The model under review builds one solid part; all positions refer to its coordinate system, in mm. A direction names the side the tool comes from. Round coordinates to 2 decimals unless told otherwise and drop trailing zeros. Order: outer loops, then holes, each group sorted by start corner. A loop starts at its lowest first (then second) coordinate and runs counter-clockwise, first axis right, second up.
```python
from build123d import *

# Parameters (mm, degrees)
PERIMETER_DEPTH      = 4.124453
PERIMETER_DEPTH_BACK = 31
SKETCH2_W            = 95.636537696
SKETCH2_H            = 63.255720718
SKETCH2_W_2          = 91.636537696
SKETCH2_H_2          = 59.255720718
USB_HOLE_START       = -66.6
SKETCH4_W            = 13.571838798
SKETCH4_H            = 8.15289322
USB_HOLE_DEPTH       = 81
BOTTOM_START         = -31
SKETCH2_12_W         = 95.636537696
SKETCH2_12_H         = 63.255720718
BOTTOM_DEPTH         = 2
SKETCH4_6_W          = 6
SKETCH4_6_H          = 2.002355377
LOCKING_HOLE_DEPTH   = 152
FILLET1_R            = 3
STRAWS_START         = -31
SKETCH2_14_R         = 2.578463196
SKETCH2_14_R_2       = 1.375
SKETCH2_14_R_3       = 2.558752615
SKETCH2_14_R_4       = 1.372691975
SKETCH2_14_R_5       = 2.568645486
SKETCH2_14_R_6       = 1.384737696
SKETCH2_14_R_7       = 2.568443666
SKETCH2_14_R_8       = 1.388555099
STRAWS_DEPTH         = 15.415068015
CUT_EXTRUDE3_START   = -68
SKETCH2_16_R         = 1.375
SKETCH2_16_R_2       = 1.388555099
SKETCH2_16_R_3       = 1.384737696
SKETCH2_16_R_4       = 1.372691975
CUT_EXTRUDE3_DEPTH   = 68


with BuildPart() as part:
    # Sketch2 → Perimeter (new, two sides: drawn at the far end of the back side and taken through both)
    with BuildSketch(Plane.XY.offset(-PERIMETER_DEPTH_BACK)):
        with Locations((147.401306837, -96.227860359)):
            Rectangle(SKETCH2_W, SKETCH2_H)
        with Locations((147.401306837, -96.227860359)):
            Rectangle(SKETCH2_W_2, SKETCH2_H_2, mode=Mode.SUBTRACT)
    extrude(amount=PERIMETER_DEPTH + PERIMETER_DEPTH_BACK)

    # Sketch4 → USB_Hole (cut)
    with BuildSketch(Plane(origin=(0, 0, 0), x_dir=(1, 0, 0), z_dir=(0, 1, 0)).offset(USB_HOLE_START)):
        with Locations((179.410729964, 14.588485375)):
            Rectangle(SKETCH4_W, SKETCH4_H)
    extrude(amount=-USB_HOLE_DEPTH, mode=Mode.SUBTRACT)

    # Sketch2<12> → Bottom (add)
    with BuildSketch(Plane.XY.offset(BOTTOM_START)):
        with Locations((147.401306837, -96.227860359)):
            Rectangle(SKETCH2_12_W, SKETCH2_12_H)
    extrude(amount=-BOTTOM_DEPTH)

    # Sketch4<6> → Locking_Hole (cut)
    with BuildSketch(Plane(origin=(0, 0, 0), x_dir=(1, 0, 0), z_dir=(0, 1, 0))):
        with Locations((131.455, 4.874369651)):
            Rectangle(SKETCH4_6_W, SKETCH4_6_H)
        with Locations((183.452691975, 4.874369651)):
            Rectangle(SKETCH4_6_W, SKETCH4_6_H)
    extrude(amount=-LOCKING_HOLE_DEPTH, mode=Mode.SUBTRACT)

    # Fillet1
    fillet1_edges = [part.edges().sort_by_distance(p)[0] for p in [
        (101.583037989, -125.855720718, -13.4377735),
        (101.583037989, -66.6, -13.4377735),
        (193.219575685, -66.6, -13.4377735),
        (195.219575685, -64.6, -14.4377735),
        (193.219575685, -125.855720718, -13.4377735),
        (195.219575685, -127.855720718, -14.4377735),
        (99.583037989, -64.6, -14.4377735),
        (99.583037989, -127.855720718, -14.4377735),
    ]]
    fillet(fillet1_edges, radius=FILLET1_R)

    # Sketch2<14> → Straws (add)
    # profile 1 of 4: a face of its own
    with BuildSketch(Plane.XY.offset(STRAWS_START)):
        with Locations(Location((128.455, -71.07, 0), (0, 0, 180))):
            Circle(SKETCH2_14_R)
        with Locations(Location((128.455, -71.07, 0), (0, 0, 180))):
            Circle(SKETCH2_14_R_2, mode=Mode.SUBTRACT)
    # profile 2 of 4: a face of its own
    with BuildSketch(Plane.XY.offset(STRAWS_START)):
        with Locations(Location((186.452691975, -71.07, 0), (0, 0, 180))):
            Circle(SKETCH2_14_R_3)
        with Locations(Location((186.452691975, -71.07, 0), (0, 0, 180))):
            Circle(SKETCH2_14_R_4, mode=Mode.SUBTRACT)
    # profile 3 of 4: a face of its own
    with BuildSketch(Plane.XY.offset(STRAWS_START)):
        with Locations(Location((128.455, -120.060262304, 0), (0, 0, 180))):
            Circle(SKETCH2_14_R_5)
        with Locations(Location((128.455, -120.060262304, 0), (0, 0, 180))):
            Circle(SKETCH2_14_R_6, mode=Mode.SUBTRACT)
    # profile 4 of 4: a face of its own
    with BuildSketch(Plane.XY.offset(STRAWS_START)):
        with Locations(Location((186.452691975, -120.060262304, 0), (0, 0, 180))):
            Circle(SKETCH2_14_R_7)
        with Locations(Location((186.452691975, -120.060262304, 0), (0, 0, 180))):
            Circle(SKETCH2_14_R_8, mode=Mode.SUBTRACT)
    extrude(amount=STRAWS_DEPTH)

    # Sketch2<16> → Cut-Extrude3 (cut)
    with BuildSketch(Plane.XY.offset(CUT_EXTRUDE3_START)):
        with Locations(Location((128.455, -71.07, 0), (0, 0, 180))):
            Circle(SKETCH2_16_R)
        with Locations(Location((186.452691975, -120.060262304, 0), (0, 0, 180))):
            Circle(SKETCH2_16_R_2)
        with Locations(Location((128.455, -120.060262304, 0), (0, 0, 180))):
            Circle(SKETCH2_16_R_3)
        with Locations(Location((186.452691975, -71.07, 0), (0, 0, 180))):
            Circle(SKETCH2_16_R_4)
    extrude(amount=CUT_EXTRUDE3_DEPTH, mode=Mode.SUBTRACT)


solid = part.part
```
(1) Consider section D-D (y = -96.5). Write out the cut boundary in (x, z), and give its area (3 significant figures).
Data:
outline: (99.58, -33) - (195.22, -33) - (195.22, 4.12) - (193.22, 4.12) - (193.22, -31) - (101.58, -31) - (101.58, 4.12) - (99.58, 4.12) - close
area: 332 mm2
(2) Consider section A-A (y = -71.07). Write out the cut boundary in (x, z), and give its area (3 significant figures).
Data:
outline: (99.58, -33) - (127.08, -33) - (127.08, -15.58) - (125.88, -15.58) - (125.88, -31) - (101.58, -31) - (101.58, 4.12) - (99.58, 4.12) - close; (129.83, -33) - (185.08, -33) - (185.08, -15.58) - (183.89, -15.58) - (183.89, -31) - (131.03, -31) - (131.03, -15.58) - (129.83, -15.58) - close; (187.83, -33) - (195.22, -33) - (195.22, 4.12) - (193.22, 4.12) - (193.22, -31) - (189.01, -31) - (189.01, -15.58) - (187.83, -15.58) - close
area: 394 mm2
(3) Consider section C-C (z = -29). State how many separate pieces and enclosed holes the cut face has, and give its area (3 significant figures).
Data:
separate pieces: 5
enclosed holes: 5
area: 679 mm2
(4) Insertion check: pin 1 (3 mm diameter, centred on x = 134, y = -79, fed in from +Z); pin 2 (1.6 mm diameter, centred on y = -66, z = -5, fed in from -X); pin 3 (2 mm diameter, centred on y = -65.5, z = -4.5, fed in from +X). Each pin has a flat end and moves straight along its axis. Give the tip position at first contact, or say it passes through.
Data:
pin 1: stops at z = -31
pin 2: stops at x = 99.69
pin 3: stops at x = 195.01
(5) Draft analysis for pull direction Z (two halves, no side actions). For faces 4 (the flat face through (127, -70, -15.585)), 5 (the flat face through (131, -66, -5.876)), 6 (the cylindrical face through (192.32, -125, -13.19)), state which applies: pulls with the +Z half, pulls with the -Z half, needs draft (parallel to the pull), parting line crosses it, or undercut.
Data:
face 4: pulls with the +Z half
face 5: undercut
face 6: needs draft
(6) Consider section B-B (z = 1). Write out the cut boundary in (x, y).
Data:
outline: (99.58, -124.86) arc R3 ccw to (102.58, -127.86) - (192.22, -127.86) arc R3 ccw to (195.22, -124.86) - (195.22, -67.6) arc R3 ccw to (192.22, -64.6) - (102.58, -64.6) arc R3 ccw to (99.58, -67.6) - close; hole (101.58, -122.86) arc R3 ccw to (104.58, -125.86) - (190.22, -125.86) arc R3 ccw to (193.22, -122.86) - (193.22, -69.6) arc R3 ccw to (190.22, -66.6) - (104.58, -66.6) arc R3 ccw to (101.58, -69.6) - close
(7) For faces 1 (the flat face through (185, -119, -15.585)), 2 (the flat face through (128.455, -127, -5)), 3 (the flat face through (179, -127, -18.665)), list the 3-axis set-ups (+Z, -Z, +X, -X, +Y, -Y) from which the entire face can be reached by the end or side of a thin tool; tool diameter is ignored.
Data:
face 1: +Z
face 2: +Y, -Y
face 3: -Y
(8) To check wall thickness, follow probe 1 along X at (y, z) = (-71.07, -20.25); probe 2 along Y at (x, z) = (169, -12.5); probe 3 along X at (y, z) = (-87.5, -9). State the ranges of each line that lie inside material, in increasing order.
Data:
probe 1: x = 99.58 to 101.58, 125.88 to 127.08, 129.83 to 131.03, 183.89 to 185.08, 187.83 to 189.01, 193.22 to 195.22
probe 2: y = -127.86 to -125.86, -66.6 to -64.6
probe 3: x = 99.58 to 101.58, 193.22 to 195.22
